For this review, use the dimensioned drawing (mm, ordinates from the lowest corner) and the shaded views. Coordinates: 2 decimals unless noted, no trailing zeros. Loops run counter-clockwise (first coordinate to the right, second up) from the corner with the lowest first, then second, coordinate; pieces in that order, holes last. Notation, with made-up numbers: (72.25, -10) - (111.25, -10) arc R18 ccw to (111.25, 9) - close; hole circle Ø8 at (-19, 38). An arc over 180 degrees is marked (long way). Answer in a Markdown table with one row per item. Add a question column.
(1) We need section B-B on x = 35.56. Write out the cut boundary in (y, z), plus the area to 3 significant figures.
(2) We need section A-A on z = 300.99. Write out the cut boundary in (x, y).
(3) For line 1 along Z through (x, y) = (35.56, 4.5); line 2 along Z through (x, y) = (42.5, 3.75), list the stretches that pass through material, from the lowest coordinate up.
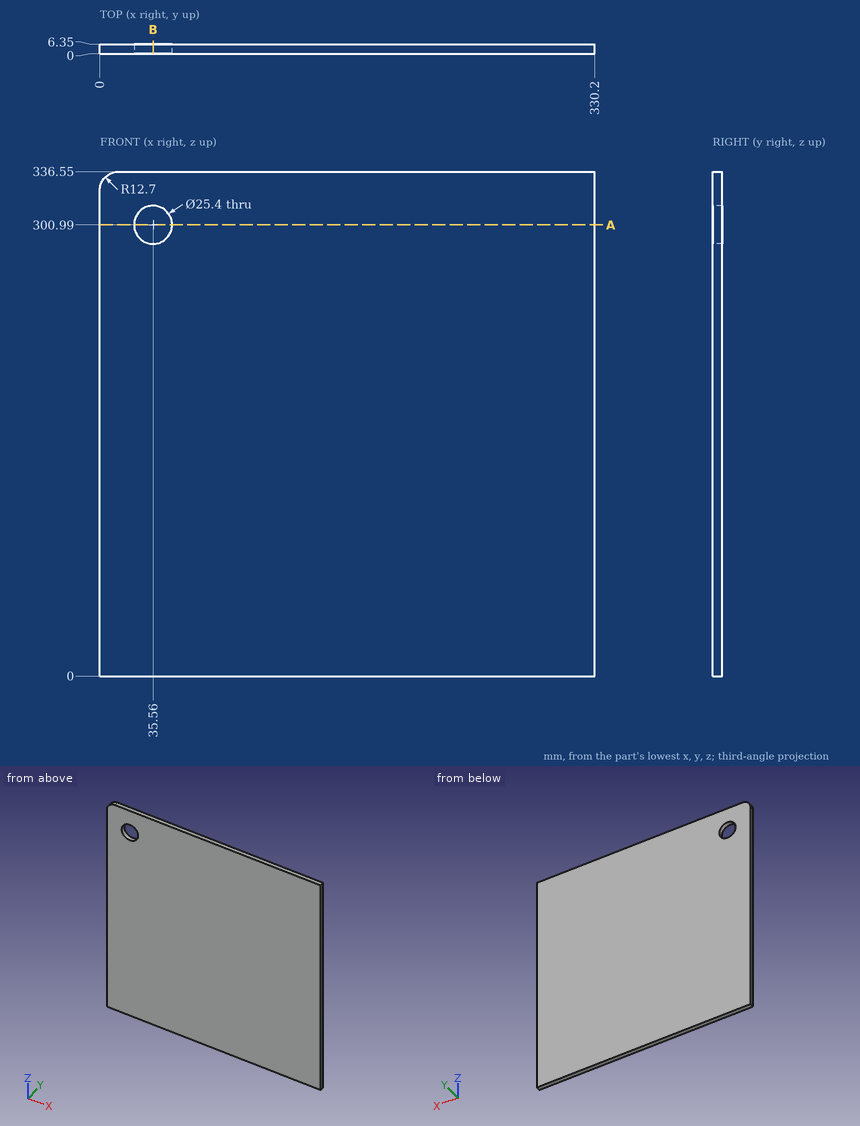
Outcome:
| question | item | result |
|---|---|---|
| 1 | outline | (0, 0) - (6.35, 0) - (6.35, 288.29) - (0, 288.29) - close; (0, 313.69) - (6.35, 313.69) - (6.35, 336.55) - (0, 336.55) - close |
| 1 | area | 1,980 mm² |
| 2 | outline | (0, 0) - (22.86, 0) - (22.86, 6.35) - (0, 6.35) - close; (48.26, 0) - (330.2, 0) - (330.2, 6.35) - (48.26, 6.35) - close |
| 3 | line 1 | 0 to 288.29, 313.69 to 336.55 |
| 3 | line 2 | 0 to 290.35, 311.63 to 336.55 |
